```python
from build123d import *

# Parameters (mm, degrees)
SKETCH2_R           = 34.599541738
SKETCH2_R_2         = 14.2875
SKETCH2_R_3         = 6.35
SKETCH2_R_4         = 3.2639
SKETCH2_R_5         = 28.329529504
BOSS_EXTRUDE2_DEPTH = 6.35


with BuildPart() as part:
    # Sketch2 → Boss-Extrude2 (new body)
    # profile 1 of 10: a face of its own
    with BuildSketch(Plane(origin=(0, 0, 0), x_dir=(0, 0, -1), z_dir=(1, 0, 0))):
        with Locations((54.99261314, -31.75)):
            Circle(SKETCH2_R)
        with Locations((54.99261314, -31.75)):
            Circle(SKETCH2_R_2, mode=Mode.SUBTRACT)
    # profile 2 of 10: a face of its own
    with BuildSketch(Plane(origin=(0, 0, 0), x_dir=(0, 0, -1), z_dir=(1, 0, 0))):
        with BuildLine():
            ThreePointArc((57.000696707, -66.291220141), (31.247618749, -56.915522641), (20.393071403, -31.75))
            Line((20.393071403, -31.75), (20.393071403, -103.183274949))
            ThreePointArc((20.393071403, -103.183274949), (26.743071403, -96.833274949), (33.093071403, -103.183274949))
            ThreePointArc((33.093071403, -103.183274949), (31.233199463, -107.67340301), (26.743071403, -109.533274949))
            Line((26.743071403, -109.533274949), (52.143071403, -109.533274949))
            ThreePointArc((52.143071403, -109.533274949), (47.652943342, -98.693146889), (58.493071403, -103.183274949))
            ThreePointArc((58.493071403, -103.183274949), (58.33576166, -104.587941235), (57.87162656, -105.923011398))
            Line((57.87162656, -105.923011398), (77.392896244, -65.105702067))
            Line((77.392896244, -65.105702067), (57.000696707, -66.291220141))
        make_face()
    # profile 3 of 10: a face of its own
    with BuildSketch(Plane(origin=(0, 0, 0), x_dir=(0, 0, -1), z_dir=(1, 0, 0))):
        with Locations((52.143071403, -103.183274949)):
            Circle(SKETCH2_R_3)
        with Locations((52.143071403, -103.183274949)):
            Circle(SKETCH2_R_4, mode=Mode.SUBTRACT)
    # profile 4 of 10: a face of its own
    with BuildSketch(Plane(origin=(0, 0, 0), x_dir=(0, 0, -1), z_dir=(1, 0, 0))):
        with Locations((26.743071403, -103.183274949)):
            Circle(SKETCH2_R_3)
        with Locations((26.743071403, -103.183274949)):
            Circle(SKETCH2_R_4, mode=Mode.SUBTRACT)
    # profile 5 of 10: a face of its own
    with BuildSketch(Plane(origin=(0, 0, 0), x_dir=(0, 0, -1), z_dir=(1, 0, 0))):
        with Locations((131.170104981, -33.601954858)):
            Circle(SKETCH2_R_5)
        with Locations((131.170104981, -33.601954858)):
            Circle(SKETCH2_R_2, mode=Mode.SUBTRACT)
    # profile 6 of 10: a face of its own
    with BuildSketch(Plane(origin=(0, 0, 0), x_dir=(0, 0, -1), z_dir=(1, 0, 0))):
        with BuildLine():
            Line((134.186655208, -5.433485487), (58.676799121, 2.652835088))
            ThreePointArc((58.676799121, 2.652835088), (80.727797568, -8.623639047), (89.592154878, -31.75))
            ThreePointArc((89.592154878, -31.75), (88.735013932, -39.403670834), (86.206059323, -46.678130018))
            Line((86.206059323, -46.678130018), (77.392896244, -65.105702067))
            Line((77.392896244, -65.105702067), (117.180043235, -62.792642027))
            Line((117.180043235, -62.792642027), (108.094917525, -50.036612316))
            ThreePointArc((108.094917525, -50.036612316), (106.717150914, -19.297575132), (134.186655208, -5.433485487))
        make_face()
    # profile 7 of 10: a face of its own
    with BuildSketch(Plane(origin=(0, 0, 0), x_dir=(0, 0, -1), z_dir=(1, 0, 0))):
        with BuildLine():
            ThreePointArc((86.206059323, -46.678130018), (74.282139722, -60.47355223), (57.000696707, -66.291220141))
            Line((57.000696707, -66.291220141), (77.392896244, -65.105702067))
            Line((77.392896244, -65.105702067), (86.206059323, -46.678130018))
        make_face()
    # profile 8 of 10: a face of its own
    with BuildSketch(Plane(origin=(0, 0, 0), x_dir=(0, 0, -1), z_dir=(1, 0, 0))):
        with BuildLine():
            ThreePointArc((132.814290418, -61.883731609), (118.926309787, -59.149004025), (108.094917525, -50.036612316))
            Line((108.094917525, -50.036612316), (117.180043235, -62.792642027))
            Line((117.180043235, -62.792642027), (132.814290418, -61.883731609))
        make_face()
    # profile 9 of 10: a face of its own
    with BuildSketch(Plane(origin=(0, 0, 0), x_dir=(0, 0, -1), z_dir=(1, 0, 0))):
        with BuildLine():
            Line((160.092841091, -103.129192537), (159.498606986, -33.360674656))
            ThreePointArc((159.498606986, -33.360674656), (159.49937761, -33.481313663), (159.499634486, -33.601954858))
            ThreePointArc((159.499634486, -33.601954858), (151.775216505, -53.043961468), (132.814290418, -61.883731609))
            Line((132.814290418, -61.883731609), (117.180043235, -62.792642027))
            Line((117.180043235, -62.792642027), (148.570820295, -106.867066268))
            ThreePointArc((148.570820295, -106.867066268), (151.78359124, -97.143164231), (160.092841091, -103.129192537))
        make_face()
    # profile 10 of 10: a face of its own
    with BuildSketch(Plane(origin=(0, 0, 0), x_dir=(0, 0, -1), z_dir=(1, 0, 0))):
        with Locations((153.743071403, -103.183274949)):
            Circle(SKETCH2_R_3)
        with Locations((153.743071403, -103.183274949)):
            Circle(SKETCH2_R_4, mode=Mode.SUBTRACT)
    extrude(amount=BOSS_EXTRUDE2_DEPTH)


solid = part.part
```
Can you work these out from the model? Positions are in its coordinate system, mm. A direction names the side the tool comes from. Round coordinates to 2 decimals unless told otherwise and drop trailing zeros. Order: outer loops, then holes, each group sorted by start corner. A loop starts at its lowest first (then second) coordinate and runs counter-clockwise, first axis right, second up. Notation, with made-up numbers: (76, -31.75) -> (115, -31.75) arc R16 ccw to (115, -1.75) -> close; hole circle Ø3 at (42.5, 75.5). An arc over 180 degrees is marked (long way). Return JSON: item names as keys, results as strings. Group by question number.
1. We'd pull the mould along Y, two halves only. Please class faces 3 (the face through (0, -40, -89)), 4 (the face through (3.131, -5.745, -32.17)), 5 (the face through (3.131, -105.169, -151.153)), 6 (the face through (3.13, -108.58, -55.49)): released by +Y, released by -Y, zero draft, split by the parting line, or undercut.
2. I need wall thicknesses on line 1 (Y direction, x = 3.25, z = -50); line 2 (Y direction, x = 1.75, z = -49.5); line 3 (Z direction, x = 2, y = -98.5). Which ranges of each line are inside material? Lowest first, please. Write a range as [from, to].
3. Which directions (+Z, -Z, +X, -X, +Y, -Y) give clear straight access to the entire face, cutting with the end or side of a thin tool? Please do faces 1 (the face through (6.35, -40, -89)), 2 (the face through (3.131, -63.965, -97.008)).
4. If we section it at B-B, the plane z = -62: Write out the boundary of the cut face in (x, y).
5. If we section it at D-D, the plane x = 1: Count the separate pieces of the cut face and the enclosed holes in it, then the cut area to 3 significant figures.
6. If we section it at C-C, the plane y = -79: Write out the boundary of the cut face in (x, z).
7. If we section it at A-A, the plane y = -39: Write out the boundary of the cut face in (x, z), then the cut area to 3 significant figures.
8. Will these pins go through, and if not, where does the flat tip stop? pin 1 (6 mm diameter, centred on y = -103.18, z = -52.14, fed in from +X); pin 2 (3 mm diameter, centred on x = 5, z = -64, fed in from -Y); pin 3 (2 mm diameter, centred on y = -16.5, z = -112.5, fed in from -X).
Output values:
{
 "1": {"face 3": "zero draft", "face 4": "released by +Y", "face 5": "undercut", "face 6": "released by -Y"},
 "2": {"line 1": "[-109.53, -105.65], [-100.72, -45.14], [-18.36, 2.49]", "line 2": "[-109.53, -105.1], [-101.27, -44.94], [-18.56, 2.41]", "line 3": "[-160.05, -142.61], [-61.42, -20.39]"},
 "3": {"face 1": "+Z, -Z, +X, +Y, -Y", "face 2": "+X, -X, -Y"},
 "4": {"outline": "(0, -97.29) -> (6.35, -97.29) -> (6.35, -44.2) -> (0, -44.2) -> close; (0, -19.3) -> (6.35, -19.3) -> (6.35, 2.3) -> (0, 2.3) -> close"},
 "5": {"separate pieces": "1", "enclosed holes": "5", "area": "10,200 mm²"},
 "6": {"outline": "(0, -159.89) -> (6.35, -159.89) -> (6.35, -128.72) -> (0, -128.72) -> close; (0, -70.75) -> (6.35, -70.75) -> (6.35, -20.39) -> (0, -20.39) -> close"},
 "7": {"outline": "(0, -159.55) -> (6.35, -159.55) -> (6.35, -144.4) -> (0, -144.4) -> close; (0, -117.94) -> (6.35, -117.94) -> (6.35, -67.3) -> (0, -67.3) -> close; (0, -42.68) -> (6.35, -42.68) -> (6.35, -20.39) -> (0, -20.39) -> close", "area": "559 mm²"},
 "8": {"pin 1": "through", "pin 2": "y = -96.25", "pin 3": "x = 0"}
}
